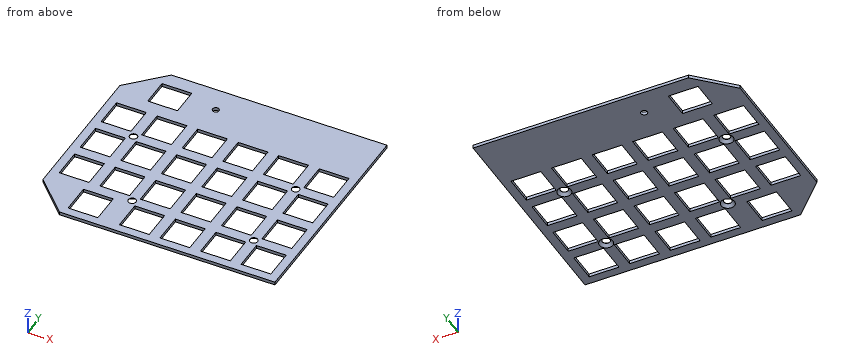
from build123d import *

# Parameters (mm, degrees)
BOSS_EXTRU_1_DEPTH                          = 1.5
ESQUISSE3_R                                 = 1.5
ESQUISSE3_W                                 = 14
ESQUISSE3_H                                 = 14
ESQUISSE3_H_2                               = 13
ENL_V_MAT_EXTRU_2_DEPTH                     = 10
FRAISAGE_POUR_VIS_T_TE_FRAIS_E_M31_AT_COUNT = 2
FRAISAGE_POUR_VIS_T_TE_FRAIS_E_M31_AT_PITCH = 38.1
FRAISAGE_POUR_VIS_T_TE_FRAIS_E_M31_2_COUNT  = 2
FRAISAGE_POUR_VIS_T_TE_FRAIS_E_M31_2_PITCH  = 76.2
FRAISAGE_POUR_VIS_T_TE_FRAIS_E_M31_3_COUNT  = 2
FRAISAGE_POUR_VIS_T_TE_FRAIS_E_M31_3_PITCH  = 68.685751798


with BuildPart() as part:
    # Esquisse1 → Boss.-Extru.1 (new body)
    with BuildSketch(Plane.XY):
        Polygon((0, -85), (16, -101), (117.25, -101), (117.25, 1), (16, 1), (0, -15), align=None)
    extrude(amount=BOSS_EXTRU_1_DEPTH)

    # Esquisse3 → Enlèv. mat.-Extru.2 (cut)
    with BuildSketch(Plane(origin=(0, 0, 0), x_dir=(-1, 0, 0), z_dir=(0, 0, -1))):
        with Locations((-43, -11)):
            Circle(ESQUISSE3_R)
        with Locations((-87.2, -32.85)):
            Rectangle(ESQUISSE3_W, ESQUISSE3_H)
        with Locations((-106.25, -32.85)):
            Rectangle(ESQUISSE3_W, ESQUISSE3_H)
        with Locations((-68.15, -32.85)):
            Rectangle(ESQUISSE3_W, ESQUISSE3_H)
        with Locations((-49.1, -32.85)):
            Rectangle(ESQUISSE3_W, ESQUISSE3_H)
        with Locations((-30.05, -32.85)):
            Rectangle(ESQUISSE3_W, ESQUISSE3_H)
        with Locations((-11, -32.85)):
            Rectangle(ESQUISSE3_W, ESQUISSE3_H)
        with Locations((-87.2, -51.9)):
            Rectangle(ESQUISSE3_W, ESQUISSE3_H)
        with Locations((-68.15, -51.9)):
            Rectangle(ESQUISSE3_W, ESQUISSE3_H)
        with Locations((-49.1, -51.9)):
            Rectangle(ESQUISSE3_W, ESQUISSE3_H)
        with Locations((-30.05, -51.9)):
            Rectangle(ESQUISSE3_W, ESQUISSE3_H)
        with Locations((-11, -51.9)):
            Rectangle(ESQUISSE3_W, ESQUISSE3_H)
        with Locations((-87.2, -70.95)):
            Rectangle(ESQUISSE3_W, ESQUISSE3_H)
        with Locations((-68.15, -70.95)):
            Rectangle(ESQUISSE3_W, ESQUISSE3_H)
        with Locations((-49.1, -70.95)):
            Rectangle(ESQUISSE3_W, ESQUISSE3_H)
        with Locations((-30.05, -70.95)):
            Rectangle(ESQUISSE3_W, ESQUISSE3_H)
        with Locations((-11, -70.95)):
            Rectangle(ESQUISSE3_W, ESQUISSE3_H)
        with Locations((-87.2, -90)):
            Rectangle(ESQUISSE3_W, ESQUISSE3_H)
        with Locations((-68.15, -90)):
            Rectangle(ESQUISSE3_W, ESQUISSE3_H)
        with Locations((-49.1, -90)):
            Rectangle(ESQUISSE3_W, ESQUISSE3_H)
        with Locations((-106.25, -51.9)):
            Rectangle(ESQUISSE3_W, ESQUISSE3_H)
        with Locations((-106.25, -70.95)):
            Rectangle(ESQUISSE3_W, ESQUISSE3_H)
        with Locations((-106.25, -90)):
            Rectangle(ESQUISSE3_W, ESQUISSE3_H)
        with Locations((-24.97, -90)):
            Rectangle(ESQUISSE3_W, ESQUISSE3_H)
        with Locations((-22.05, -12.35)):
            Rectangle(ESQUISSE3_W, ESQUISSE3_H_2)
    extrude(amount=-ENL_V_MAT_EXTRU_2_DEPTH, mode=Mode.SUBTRACT)

    # Esquisse6 → Fraisage pour vis à tête fraisée M31 (revolve, cut)
    with BuildSketch(Plane(origin=(96.725, -42.375, 0), x_dir=(0, 1, 0), z_dir=(1, 0, 0))):
        Polygon((0, 0), (0, 1.5), (1.8, 1.5), (1.8, 1.35), (3.15, 0), align=None)
    fraisage_pour_vis_t_te_frais_e_m31 = revolve(axis=Axis((96.725, -42.375, -6.35), (0, 0, 1)), mode=Mode.SUBTRACT)

    # Fraisage pour vis à tête fraisée M31 at: Fraisage pour vis à tête fraisée M31 ×2
    with Locations(*[(0, -i * FRAISAGE_POUR_VIS_T_TE_FRAIS_E_M31_AT_PITCH, 0) for i in range(1, FRAISAGE_POUR_VIS_T_TE_FRAIS_E_M31_AT_COUNT)]):
        add(fraisage_pour_vis_t_te_frais_e_m31, mode=Mode.SUBTRACT)

    # Fraisage pour vis _ t_te frais_e M31 2: Fraisage pour vis à tête fraisée M31 ×2
    with Locations(*[(-i * FRAISAGE_POUR_VIS_T_TE_FRAIS_E_M31_2_PITCH, 0, 0) for i in range(1, FRAISAGE_POUR_VIS_T_TE_FRAIS_E_M31_2_COUNT)]):
        add(fraisage_pour_vis_t_te_frais_e_m31, mode=Mode.SUBTRACT)

    # Fraisage pour vis _ t_te frais_e M31 3: Fraisage pour vis à tête fraisée M31 ×2
    with Locations(*[Vector(-0.832050294, -0.554700196, 0) * (i * FRAISAGE_POUR_VIS_T_TE_FRAIS_E_M31_3_PITCH) for i in range(1, FRAISAGE_POUR_VIS_T_TE_FRAIS_E_M31_3_COUNT)]):
        add(fraisage_pour_vis_t_te_frais_e_m31, mode=Mode.SUBTRACT)


solid = part.part
Work out the finished part from the listing and answer in its coordinate system (mm). Give positions to 0.01 mm unless a question says otherwise; leave off trailing zeros. Loops run counter-clockwise (first coordinate to the right, second up) from the corner with the lowest first, then second, coordinate; pieces in that order, holes last. Notation, with made-up numbers: M 69,86 L 86,86 A23 ccw 86,114 Z; hole C -25,16.25 d11. An arc over 180 degrees is marked long. Use CSV: the item, a comma, the result in double quotes.
1) Consider L1, parallel to Y at x = 33, z = 0.2; L2, parallel to Y at x = 73, z = 0.85; L3, parallel to X at y = -83.5, z = 0.2. Determine where each line is inside the solid, lowest interval first.
Answer:
L1,"-101 to -77.95, -63.95 to -58.9, -44.9 to -39.85, -25.85 to 1"
L2,"-101 to -97, -83 to -77.95, -63.95 to -58.9, -44.9 to -39.85, -25.85 to 1"
L3,"0 to 17.97, 31.97 to 42.1, 56.1 to 61.15, 75.15 to 80.2, 94.2 to 99.25, 113.25 to 117.25"
2) Find section C-C on x = 67. Write down the section's boundary in (y, z), plus the area to 3 significant figures.
Answer:
outline,"M -101,0 L -97,0 L -97,1.5 L -101,1.5 Z; M -83,0 L -77.95,0 L -77.95,1.5 L -83,1.5 Z; M -63.95,0 L -58.9,0 L -58.9,1.5 L -63.95,1.5 Z; M -44.9,0 L -39.85,0 L -39.85,1.5 L -44.9,1.5 Z; M -25.85,0 L 1,0 L 1,1.5 L -25.85,1.5 Z"
area,"69.0 mm^2"
3) Find section B-B on x = 12. Write down the section's boundary in (y, z).
Answer:
outline,"M -97,0 L -77.95,0 L -77.95,1.5 L -97,1.5 Z; M -63.95,0 L -58.9,0 L -58.9,1.5 L -63.95,1.5 Z; M -44.9,0 L -39.85,0 L -39.85,1.5 L -44.9,1.5 Z; M -25.85,0 L -3,0 L -3,1.5 L -25.85,1.5 Z"
4) Given P1, Ø0.8, axis at y = -91.5, z = 0.5, coming from the -X side, flat-ended and moving along its own axis, determine where the tip first touches the part or whether it passes through.
Answer:
P1,"x = 6.1"
5) Find section D-D on y = -68. Write down the section's boundary in (x, z).
Answer:
outline,"M 0,0 L 4,0 L 4,1.5 L 0,1.5 Z; M 18,0 L 23.05,0 L 23.05,1.5 L 18,1.5 Z; M 37.05,0 L 42.1,0 L 42.1,1.5 L 37.05,1.5 Z; M 56.1,0 L 61.15,0 L 61.15,1.5 L 56.1,1.5 Z; M 75.15,0 L 80.2,0 L 80.2,1.5 L 75.15,1.5 Z; M 94.2,0 L 99.25,0 L 99.25,1.5 L 94.2,1.5 Z; M 113.25,0 L 117.25,0 L 117.25,1.5 L 113.25,1.5 Z"
6) Find section A-A on y = -11. Write down the section's boundary in (x, z), plus the area to 3 significant figures.
Answer:
outline,"M 4,0 L 15.05,0 L 15.05,1.5 L 4,1.5 Z; M 29.05,0 L 41.5,0 L 41.5,1.5 L 29.05,1.5 Z; M 44.5,0 L 117.25,0 L 117.25,1.5 L 44.5,1.5 Z"
area,"144 mm^2"
